Part model, mm, in its own coordinate system. A direction names the side the tool comes from. Give positions to 0.01 mm unless a question says otherwise; leave off trailing zeros. Order: outer loops, then holes, each group sorted by start corner. A loop starts at its lowest first (then second) coordinate and runs counter-clockwise, first axis right, second up. Notation, with made-up numbers: M 85.5,25 L 106.5,25 A18 ccw 106.5,52 Z; hole C -23.75,71.25 d4. An arc over 180 degrees is marked long. One line per question, with ' | ' between items.
Autodesk Inventor part; units mm, degrees
ref_plane "YZ Plane" through (0, 0, 0) normal (1, 0, 0) x (0, 1, 0)
ref_plane "XZ Plane" through (0, 0, 0) normal (0, 1, 0) x (-1, 0, 0)
ref_plane "XY Plane" through (0, 0, 0) normal (0, 0, 1) x (1, 0, 0)
sketch "Sketch1" plane through (0, 0, 0) normal (0, 0, 1) x (1, 0, 0)
  line L0 (0, 0) -> (44.45, 0)
  line L1 (44.45, 0) -> (44.45, 98)
  line L2 (44.45, 98) -> (0, 98)
  line L3 (0, 98) -> (0, 0)
  line L4 (4.7625, 0) -> (0, 0)
  line L5 (0, 0) -> (0, -35)
  line L6 (0, -35) -> (4.7625, -35)
  line L7 (4.7625, -35) -> (4.7625, 0)
  line L8 (4.7625, -35) -> (12.7, -35)
  line L9 (12.7, -35) -> (12.7, 0)
  line L10 (12.7, 0) -> (4.7625, 0)
  line L11 (4.7625, 0) -> (4.7625, -35)
  line L12 (0, 98) -> (52.5, 98)
  line L13 (52.5, 98) -> (52.5, 168)
  line L14 (52.5, 168) -> (0, 168)
  line L15 (0, 168) -> (0, 98)
  dimension "d0" = 44.45
  dimension "d1" = 98
  dimension "d3" = 4.7625
  dimension "d4" = 35
  dimension "d5" = 12.7
  dimension "d6" = 52.5
  dimension "d7" = 70
revolve "Revolution1" add sketch "Sketch1" angle 360 about axis through (0, 98, 0) along (0, -1, 0) contours L3 L2 L1 L0 | L0 L9 L8 L7 | L15 L14 L13 L12 L2
properties part number "Spindle"
1. Mould opens along X. For faces 1 (the cylindrical face through (-2.75, -17.26, 12.4)), 2 (the flat face through (-43, 98, 12)), 3 (the cylindrical face through (-3.78, -17.26, 2.9)) say: released by +X, released by -X, zero draft, split by the parting line, or undercut.
Worked out:
face 1: split by the parting line | face 2: zero draft | face 3: undercut
2. Slice it at A-A on z = 0. Give the cut face in (x, y).
Worked out:
outline: M -52.5,98 L -44.45,98 L -44.45,0 L -12.7,0 L -12.7,-35 L -4.76,-35 L -4.76,0 L 4.76,0 L 4.76,-35 L 12.7,-35 L 12.7,0 L 44.45,0 L 44.45,98 L 52.5,98 L 52.5,168 L -52.5,168 Z
3. Probe L1, parallel to Z at x = 0, y = -12.5; L2, parallel to Y at x = 17, z = -41; L3, parallel to Y at x = 22.5, z = -39. List the from-to ranges inside material, lowest first. Write a range as from..to.
Worked out:
L1: z = -12.7..-4.76, 4.76..12.7 | L2: y = 0..168 | L3: y = 98..168
4. Slice it at B-B on x = 0. Give the cut face in (y, z).
Worked out:
outline: M -35,-12.7 L 0,-12.7 L 0,-44.45 L 98,-44.45 L 98,-52.5 L 168,-52.5 L 168,52.5 L 98,52.5 L 98,44.45 L 0,44.45 L 0,12.7 L -35,12.7 L -35,4.76 L 0,4.76 L 0,-4.76 L -35,-4.76 Z
5. Slice it at C-C on y = -3. Give the cut face in (x, z) (1 decimal).
Worked out:
outline: C 0,0 d25.4; hole C 0,0 d9.5
6. Slice it at D-D on y = 33.5. Give the cut face in (x, z).
Worked out:
outline: C 0,0 d88.9
7. Drop flat-ended pins along their axis: pin 1 (8 mm diameter, centred on x = -3, y = -5.5, fed in from -Z); pin 2 (6 mm diameter, centred on y = 65.5, z = -13.5, fed in from +X); pin 3 (3 mm diameter, centred on x = 8, y = 123.5, fed in from -Z). Give the stop position or say it passes through.
Worked out:
pin 1: stops at z = -12.7 | pin 2: stops at x = 43.19 | pin 3: stops at z = -52.1
8. Tool access for faces 4 (the cylindrical face through (42.397, 49.686, -13.352)), 5 (the flat face through (-1, 168, 1)): list every direction of +Z, -Z, +X, -X, +Y, -Y with a clear straight run to the whole face (end or side of a thin tool).
Worked out:
face 4: -Y | face 5: +Z, -Z, +X, -X, +Y
